```python
from build123d import *

# Parameters (mm, degrees)
SKETCH1_W               = 66.04
SKETCH1_H               = 35.56
SKETCH1_R               = 6.35
SKETCH1_R_2             = 3.175
BOSS_EXTRUDE1_DEPTH     = 35.56
CUT_EXTRUDE1_DEPTH      = 12.7
CUT_EXTRUDE1_DEPTH_BACK = 12.7
SKETCH3_W               = 25.4
SKETCH3_H               = 25.4
CUT_EXTRUDE2_DEPTH      = 33.02
FILLET1_R               = 17.78
FILLET2_R               = 2.54


with BuildPart() as part:
    # Sketch1 → Boss-Extrude1 (new body)
    with BuildSketch(Plane.XY):
        with Locations((-15.24, 0)):
            Rectangle(SKETCH1_W, SKETCH1_H)
        Circle(SKETCH1_R, mode=Mode.SUBTRACT)
        with Locations((-35.56, 0)):
            Circle(SKETCH1_R_2, mode=Mode.SUBTRACT)
        with Locations((-22.86, 0)):
            Circle(SKETCH1_R_2, mode=Mode.SUBTRACT)
    extrude(amount=BOSS_EXTRUDE1_DEPTH)

    # Sketch2 → Cut-Extrude1 (cut, two sides)
    with BuildSketch(Plane.XY.offset(17.78)) as cut_extrude1_sk:
        with BuildLine():
            Line((0, 12.7), (17.78, 12.7))
            Line((17.78, 12.7), (17.78, -17.78))
            Line((17.78, -17.78), (-12.7, -17.78))
            Line((-12.7, -17.78), (-12.7, 0))
            ThreePointArc((-12.7, 0), (-8.980256121, 8.980256121), (0, 12.7))
        make_face()
    extrude(amount=CUT_EXTRUDE1_DEPTH, mode=Mode.SUBTRACT)
    extrude(cut_extrude1_sk.sketch, amount=-CUT_EXTRUDE1_DEPTH_BACK, mode=Mode.SUBTRACT)

    # Sketch3 → Cut-Extrude2 (cut)
    with BuildSketch(Plane.ZY.offset(48.26)):
        with Locations((17.78, 0)):
            Rectangle(SKETCH3_W, SKETCH3_H)
    extrude(amount=-CUT_EXTRUDE2_DEPTH, mode=Mode.SUBTRACT)

    # Fillet1
    fillet1_edges = [part.edges().sort_by_distance(p)[0] for p in [
        (17.78, -17.78, 2.54),
        (17.78, -17.78, 33.02),
    ]]
    fillet(fillet1_edges, radius=FILLET1_R)

    # Fillet2
    fillet2_edges = [part.edges().sort_by_distance(p)[0] for p in [
        (-24.13, -17.78, 35.56),
        (-15.24, 17.78, 35.56),
        (-24.13, -17.78, 0),
        (-48.26, 0, 0),
        (-15.24, 17.78, 0),
        (17.78, 8.89, 0),
        (17.78, 8.89, 35.56),
        (12.572358569, -12.572358569, 35.56),
        (12.572358569, -12.572358569, 0),
        (-48.26, -17.78, 17.78),
        (-48.26, 17.78, 17.78),
        (-48.26, 0, 35.56),
    ]]
    fillet(fillet2_edges, radius=FILLET2_R)


solid = part.part
```
Check sheet for the modelled part. Datum: model origin and axes. Units: mm. A direction names the side the tool comes from. Give positions to 0.01 mm unless a question says otherwise; leave off trailing zeros. Write each loop counter-clockwise with the first axis right and the second up, starting at its lowest first coordinate (ties: lowest second). Pieces come first, ordered by that corner, then holes. Notation, with made-up numbers: (-9.5, 50) - (49.5, 50) arc R15 ccw to (49.5, 64) - close; hole circle Ø1 at (21, 79.25). An arc over 180 degrees is marked (long way). Answer as a JSON object with one key per item and string values. Group by question number.
1) Sectioned sample at B-B (x = -17). Record the cut outline in (y, z), then the cut area to 3 significant figures.
2) Sectioned sample at D-D (y = 11.5). Record the cut outline in (x, z).
3) Sectioned sample at A-A (x = -35.56). Record the cut outline in (y, z) (3 decimals), then the cut area to 3 significant figures.
4) Sectioned sample at C-C (z = 22). Record the cut outline in (x, y), then the cut area to 3 significant figures.
5) Depth check by flat-ended pin: P1, Ø14, axis at y = -7.5, z = 16.5, coming from the +X side; P2, Ø4, axis at x = -22.86, y = 0, coming from the +Z side; P3, Ø5.5, axis at x = 7.5, z = 19, coming from the -Y side. Enter the tip coordinate at first touch or a pass-through.
6) Access from +Z, -Z, +X, -X, +Y, -Y to the whole of each face (thin tool, end or side, straight path). Record for faces 1 (the face through (9, 12.7, 18)), 2 (the face through (-14, 17.78, 18)).
7) Thickness scan on probe 1 along X at (y, z) = (0, 3) (3 decimals); probe 2 along X at (y, z) = (0, 1) (3 decimals); probe 3 along Y at (x, z) = (-29, 5.5). Record the ranges inside material, lowest first. Write a range as from..to.
8) Release check for a two-part mould opening along Z. For faces 3 (the face through (-48.26, 0, 31)), 4 (the face through (-32, 0, 30.48)), 5 (the face through (-32, -12.7, 18)), 6 (the face through (-22.54, -17.056, 34.796)) record: pulls with the +Z half, pulls with the -Z half, needs draft (parallel to the pull), parting line crosses it, or undercut.
Geometry results:
{
 "1": {"outline": "(-17.78, 2.54) arc R2.54 ccw to (-15.24, 0) - (15.24, 0) arc R2.54 ccw to (17.78, 2.54) - (17.78, 33.02) arc R2.54 ccw to (15.24, 35.56) - (-15.24, 35.56) arc R2.54 ccw to (-17.78, 33.02) - close; hole (-12.7, 5.08) - (12.7, 5.08) - (12.7, 30.48) - (-12.7, 30.48) - close", "area": "614 mm^2"},
 "2": {"outline": "(-48.26, 2.54) arc R2.54 ccw to (-45.72, 0) - (15.24, 0) arc R2.54 ccw to (17.78, 2.54) - (17.78, 5.08) - (-5.39, 5.08) - (-5.39, 30.48) - (17.78, 30.48) - (17.78, 33.02) arc R2.54 ccw to (15.24, 35.56) - (-45.72, 35.56) arc R2.54 ccw to (-48.26, 33.02) - (-48.26, 30.48) - (-15.24, 30.48) - (-15.24, 5.08) - (-48.26, 5.08) - close"},
 "3": {"outline": "(-17.78, 2.54) arc R2.54 ccw to (-15.24, 0) - (-3.175, 0) - (-3.175, 5.08) - (-12.7, 5.08) - (-12.7, 30.48) - (-3.175, 30.48) - (-3.175, 35.56) - (-15.24, 35.56) arc R2.54 ccw to (-17.78, 33.02) - close; (3.175, 0) - (15.24, 0) arc R2.54 ccw to (17.78, 2.54) - (17.78, 33.02) arc R2.54 ccw to (15.24, 35.56) - (3.175, 35.56) - (3.175, 30.48) - (12.7, 30.48) - (12.7, 5.08) - (3.175, 5.08) - close", "area": "549 mm^2"},
 "4": {"outline": "(-48.26, -15.24) arc R2.54 ccw to (-45.72, -17.78) - (-12.7, -17.78) - (-12.7, 0) arc R12.7 cw to (0, 12.7) - (17.78, 12.7) - (17.78, 17.78) - (-45.72, 17.78) arc R2.54 ccw to (-48.26, 15.24) - (-48.26, 12.7) - (-15.24, 12.7) - (-15.24, -12.7) - (-48.26, -12.7) - close", "area": "612 mm^2"},
 "5": {"P1": "stops at x = -12.7", "P2": "passes through", "P3": "stops at y = 12.7"},
 "6": {"face 1": "+X, -Y", "face 2": "+Z, -Z, +X, -X, +Y"},
 "7": {"probe 1": "x = -48.26..-38.735, -32.385..-26.035, -19.685..-6.35, 6.35..17.78", "probe 2": "x = -47.74..-38.735, -32.385..-26.035, -19.685..-6.35, 6.35..17.26", "probe 3": "y = -17.78..-12.7, 12.7..17.78"},
 "8": {"face 3": "needs draft", "face 4": "undercut", "face 5": "undercut", "face 6": "pulls with the +Z half"}
}
